from build123d import *

# Parameters (mm, degrees)
F0_R     = 8
F0_W     = 11
F0_H     = 32
F1_DEPTH = 11
F2_DEPTH = 9
F4_R     = 9
F5_DEPTH = 32
F6_SIZE  = 1
F7_R     = 2


with BuildPart() as f1:
    # F0 (on Front) → F1 (new body)
    with BuildSketch(Plane.XZ):
        with BuildLine():
            Line((-36, 0), (-11, 0))
            Line((-11, 0), (-11, 32))
            Line((-11, 32), (-36, 32))
            ThreePointArc((-36, 32), (-52, 16), (-36, 0))
        make_face()
        with Locations((-36, 16)):
            Circle(F0_R, mode=Mode.SUBTRACT)
        with Locations((-5.5, 16)):
            Rectangle(F0_W, F0_H)
    extrude(amount=F1_DEPTH)

    # F0 (on Front) → F2 (join)
    with BuildSketch(Plane.XZ):
        with Locations((-5.5, 16)):
            Rectangle(F0_W, F0_H)
    extrude(amount=-F2_DEPTH)

    # F3: F1 across face


with BuildPart() as f1_1:
    add(f1.part)
    add(f1.part.mirror(Plane(origin=(-5.5, 9, 16), x_dir=(1, 0, 0), z_dir=(0, 1, 0))))

    # F4 (on face) → F5 (join)
    with BuildSketch(Plane.YZ):
        with Locations((9, 16)):
            Circle(F4_R)
    extrude(amount=F5_DEPTH)

    # F6
    f6_edges = [f1_1.edges().sort_by_distance(p)[0] for p in [
        (-28, -5.5, 16),
        (-44, 0, 16),
        (-44, -11, 16),
        (-28, 23.5, 16),
        (-44, 18, 16),
        (-44, 29, 16),
    ]]
    chamfer(f6_edges, length=F6_SIZE)

    # F7
    f7_edges = [f1_1.edges().sort_by_distance(p)[0] for p in [
        (-18, -11, 32),
        (-36, -5.5, 32),
        (-23.5, 0, 32),
        (-11, 9, 32),
        (-23.5, 18, 32),
        (-36, 23.5, 32),
        (-18, 29, 32),
        (0, 9, 32),
        (-36, -5.5, 0),
        (-18, -11, 0),
        (0, 9, 0),
        (-18, 29, 0),
        (-36, 23.5, 0),
        (-23.5, 18, 0),
        (-11, 9, 0),
        (-23.5, 0, 0),
        (32, 0, 16),
        (0, 29, 16),
        (0, -11, 16),
    ]]
    fillet(f7_edges, radius=F7_R)


solid = f1_1.part
Input: part model. Units: mm. Frame: model coordinates. A direction names the side the tool comes from. Give positions to 0.01 mm unless a question says otherwise; leave off trailing zeros. Loops run counter-clockwise (first coordinate to the right, second up) from the corner with the lowest first, then second, coordinate; pieces in that order, holes last. Notation, with made-up numbers: (72.5, 50) -> (82.5, 50) arc R12 ccw to (82.5, 56) -> close; hole circle Ø5 at (74, -40). An arc over 180 degrees is marked (long way). Answer as a JSON object with one key per item and string values. Group by question number.
Item 1: Cut plane C-C, the plane z = 14.5. State how many separate pieces and enclosed holes the cut face has, and give its area (3 significant figures).
Item 2: Line query: probe 1 along Z at (x, y) = (-36, 24); probe 2 along X at (y, z) = (-8, 16.5); probe 3 along Y at (x, z) = (-48, 23.5). Output: solid intervals per line, ascending.
Item 3: Cut plane D-D, the plane x = 15.5. Return the cut outline in (y, z).
Item 4: Cut plane B-B, the plane y = 9. Return the cut outline in (x, z).
Item 5: Cut plane A-A, the plane x = -22. Return the cut outline in (y, z), and give its area (3 significant figures).
Item 6: Pin query (flat end, axial travel): P1, Ø10, axis at x = 8, y = 14, coming from the +Z side; P2, Ø2, axis at y = 5, z = 28, coming from the -X side; P3, Ø13, axis at x = -36, z = 16, coming from the -Y side; P4, Ø1, axis at x = 14.5, z = 15, coming from the +Y side. Return the tip coordinate at first contact, or that it passes through.
Item 7: Reachability of faces 1 (the cylindrical face through (-22.31, -0.57, 0.6)), 2 (the cylindrical face through (14.79, 17.584, 18.703)), 3 (the cylindrical face through (-0.57, 28.4, 16.2)) from +Z, -Z, +X, -X, +Y, -Y: full face, straight path, thin tool, end or side. Return the list, or none.
Item 8: Pull-direction query (Y, two-part tool) for faces 4 (the cylindrical face through (-22.69, 18.6, 31.43)), 5 (the cylindrical face through (-0.6, 9.25, 31.43)), 6 (the flat face through (-26, 18, 16)), 7 (the flat face through (-21, 29, 16)); classes: released by +Y, released by -Y, zero draft, split by the parting line, or undercut.
Checks:
{
 "1": {"separate pieces": "3", "enclosed holes": "0", "area": "1,550 mm²"},
 "2": {"probe 1": "z = 0 to 8, 24 to 32", "probe 2": "x = -51.99 to -43.98, -28.02 to 0", "probe 3": "y = -10.99 to -0.01, 18.01 to 28.99"},
 "3": {"outline": "circle Ø18 at (9, 16)"},
 "4": {"outline": "(-11, 2) arc R2 ccw to (-9, 0) -> (-2, 0) arc R2 ccw to (0, 2) -> (0, 7) -> (30, 7) arc R2 ccw to (32, 9) -> (32, 23) arc R2 ccw to (30, 25) -> (0, 25) -> (0, 30) arc R2 ccw to (-2, 32) -> (-9, 32) arc R2 ccw to (-11, 30) -> close"},
 "5": {"outline": "(-11, 2) arc R2 ccw to (-9, 0) -> (-2, 0) arc R2 ccw to (0, 2) -> (0, 30) arc R2 ccw to (-2, 32) -> (-9, 32) arc R2 ccw to (-11, 30) -> close; (18, 2) arc R2 ccw to (20, 0) -> (27, 0) arc R2 ccw to (29, 2) -> (29, 30) arc R2 ccw to (27, 32) -> (20, 32) arc R2 ccw to (18, 30) -> close", "area": "697 mm²"},
 "6": {"P1": "stops at z = 25", "P2": "stops at x = -11", "P3": "passes through", "P4": "stops at y = 17.99"},
 "7": {"face 1": "-Z, -X", "face 2": "+X", "face 3": "+Z, -Z, +X, +Y"},
 "8": {"face 4": "undercut", "face 5": "zero draft", "face 6": "undercut", "face 7": "released by +Y"}
}
